Autodesk Inventor part; units mm, degrees
ref_plane "YZ Plane" through (0, 0, 0) normal (1, 0, 0) x (0, 1, 0)
ref_plane "XZ Plane" through (0, 0, 0) normal (0, 1, 0) x (-1, 0, 0)
ref_plane "XY Plane" through (0, 0, 0) normal (0, 0, 1) x (1, 0, 0)
sketch "Sketch1" plane through (0, 0, 0) normal (0, 1, 0) x (-1, 0, 0)
  line L0 (0, 0) -> (60, 0)
  line L1 (55.02, -23.5) -> (55.02, -51.5)
  line L2 (60, -75) -> (0, -75)
  line L3 (0, -75) -> (0, 0)
  line L4 (55.02, -23.5) -> (72.02, -23.5) construction
  line L5 (72.02, -23.5) -> (72.02, -51.5) construction
  line L6 (72.02, -51.5) -> (55.02, -51.5) construction
  line L7 (55.02, -51.5) -> (55.02, -23.5)
  line L8 (72.02, -51.5) -> (55.02, -51.5)
  line L9 (60, -75) -> (72.02, -75)
  line L10 (72.02, -75) -> (72.02, -51.5)
  line L11 (72.02, -23.5) -> (55.02, -23.5)
  line L12 (60, 0) -> (72.02, 0)
  line L13 (72.02, 0) -> (72.02, -23.5)
  point P0 (55.02, -37.5)
  point P1 (63.52, -51.5)
  point P2 (63.52, -51.5)
  dimension "d2" = 28
  dimension "d25" = 8.5
  dimension "d26" = 60
  dimension "d27" = 12.02
  dimension "d28" = 72.02
extrude "Extrusion1" add sketch "Sketch1" along normal blind 11.8
sketch "Sketch2" plane through (-55.02, 0, -23.5) normal (0, 0, -1) x (-1, 0, 0)
  circle A0 centre (10.99, 5.9) radius 2
  line L0 (17, 0) -> (17, 11.8)
  point P0 (-55.02, 0)
  dimension "d6" = 4
  dimension "d7" = 6.01
extrude "Extrusion2" cut sketch "Sketch2" against normal blind 2
sketch "Sketch3" plane through (-72.02, 0, -51.5) normal (0, 0, 1) x (1, 0, 0)
  arc A0 (6.01, 2.2893) -> (6.0025, 9.4893) centre (6.01, 5.8893) ccw
  line L0 (0, 0) -> (0, 11.8)
  line L1 (6.01, 5.8893) -> (0, 5.9) construction
  line L2 (6.0025, 9.4893) -> (0, 9.4893)
  line L3 (6.01, 2.2893) -> (0, 2.2893)
  point P0 (72.02, 0)
  point P1 (0, 9.1893)
  point P2 (0, 2.5893)
  dimension "d10" = 7.2
  dimension "d21" = 6.01
extrude "Extrusion3" cut sketch "Sketch3" against normal blind 3.65
sketch "Sketch4" plane through (-72.02, 0, -75) normal (-1, 0, 0) x (0, 0, 1)
  line L0 (19.85, 10.7643) -> (17.45, 10.7643)
  line L1 (17.45, 10.7643) -> (17.45, 1.0143)
  line L2 (17.45, 1.0143) -> (19.85, 1.0143)
  line L3 (19.85, 1.0143) -> (19.85, 10.7643)
  line L4 (19.85, 2.2893) -> (19.85, 9.4893)
  point P0 (75, 0)
  point P1 (19.85, 5.8893)
  point P2 (19.85, 2.5893)
  point P3 (19.85, 9.1893)
  dimension "d13" = 2.4
  dimension "d14" = 9.75
extrude "Extrusion4" cut sketch "Sketch4" against normal blind 10.925
sketch "Sketch5" plane through (-72.02, 0, 0) normal (0, 0, 1) x (1, 0, 0)
  line L0 (17, 0) -> (17, 11.8)
  line L1 (72.02, 11.8) -> (0, 11.8)
  line L2 (0, 0) -> (72.02, 0)
  line L3 (17, 11.8) -> (72.02, 0)
  line L4 (72.02, 0) -> (72.02, 11.8)
  line L5 (17, 11.8) -> (72.02, 11.8)
extrude "Extrusion5" cut sketch "Sketch5" against normal blind 88.5 contours L1 L4 L3
sketch "Sketch6" plane through (-72.02, 0, -75) normal (0, 0, -1) x (-1, 0, 0)
  line L0 (0, 11.8) -> (-17, 11.8)
  line L1 (-17, 11.8) -> (-72.02, 0)
  line L2 (0, 0) -> (-72.02, 0)
  line L3 (-72.02, 0) -> (0, 0)
  line L4 (0, 11.8) -> (-17, 11.8)
  line L5 (0, 0) -> (0, 11.8)
  line L6 (-17, 0) -> (-17, 11.8)
  line L7 (0, 11.8) -> (-17, 11.8)
  line L8 (-17, 11.8) -> (-72.02, 0)
extrude "Extrusion6" add sketch "Sketch6" along normal blind 10
properties part number "hand_left_1"
Could you check a few things on this model? Use its own coordinates, in mm. A direction names the side the tool comes from. Give positions to 0.01 mm unless a question says otherwise; leave off trailing zeros. Order: outer loops, then holes, each group sorted by start corner. A loop starts at its lowest first (then second) coordinate and runs counter-clockwise, first axis right, second up.
1. Suppose I cut it at B-B (z = -69.5). List the corners of the cut face in (x, y) for me, plus the area to 3 significant figures.
2. Will these pins go through, and if not, where does the flat tip stop? P1, Ø1.2, axis at x = -66.5, z = -56.5, coming from the -Y side; P2, Ø10, axis at x = -29, z = -53, coming from the +Y side; P3, Ø8, axis at x = -37.5, z = -48.5, coming from the +Y side; P4, Ø2.5, axis at y = 5, z = -56, coming from the -X side.
3. I need wall thicknesses on L1, parallel to Z at x = -61.5, y = 6; L2, parallel to Y at x = -66, z = -22; L3, parallel to Z at x = -57.5, y = 7. Which ranges of each line are inside material? Lowest first, please.
4. Suppose I cut it at C-C (x = -28). List the corners of the cut face in (y, z) for me, plus the area to 3 significant figures.
5. For faces 1 (the flat face through (-63, 11.8, -12)), 2 (the flat face through (-67, 1.014, -56)), 3 (the flat face through (-63.6, 5.8, -23.5)), 4 (the cylindrical face through (-67.918, 6.501, -22.514)), which set-ups out of +Z, -Z, +X, -X, +Y, -Y let a thin tool reach every point of the face, with its end or its side?
6. Suppose I cut it at A-A (y = 5.9). List the corners of the cut face in (x, z) for me (3 decimals).
7. Suppose I cut it at D-D (z = -31.5). List the corners of the cut face in (x, y) for me.
8. We'd pull the mould along Y, two halves only. Please class faces 5 (the flat face through (-36, 0, -42)), 6 (the flat face through (-69, 9.489, -53)), 7 (the flat face through (-55.02, 6, -37)): pulls with the +Y half, pulls with the -Y half, needs draft (parallel to the pull), parting line crosses it, or undercut.
Solved:
1. outline: (-72.02, 0) - (0, 0) - (-55.02, 11.8) - (-72.02, 11.8) - close
1. area: 525 mm2
2. P1: stops at y = 0
2. P2: stops at y = 7.29
2. P3: stops at y = 8.9
2. P4: stops at x = -62.9
3. L1: z = -85 to -57.55, -55.15 to -51.5, -23.5 to 0
3. L2: y = 0 to 3.9, 7.9 to 11.8
3. L3: z = -85 to -51.5, -23.5 to 0
4. outline: (0, -85) - (6.01, -85) - (6.01, 0) - (0, 0) - close
4. area: 510 mm2
5. face 1: +Z, -Z, +X, -X, +Y
5. face 2: -X
5. face 3: -X, +Y, -Y
5. face 4: none
6. outline: (-72.02, -85) - (-27.51, -85) - (-27.51, 0) - (-72.02, 0) - (-72.02, -23.5) - (-68.01, -23.5) - (-68.01, -21.5) - (-64.01, -21.5) - (-64.01, -23.5) - (-55.02, -23.5) - (-55.02, -51.5) - (-62.41, -51.5) - (-62.41, -55.15) - (-61.095, -55.15) - (-61.095, -57.55) - (-72.02, -57.55) - close
7. outline: (-55.02, 0) - (0, 0) - (-55.02, 11.8) - close
8. face 5: pulls with the -Y half
8. face 6: undercut
8. face 7: needs draft
